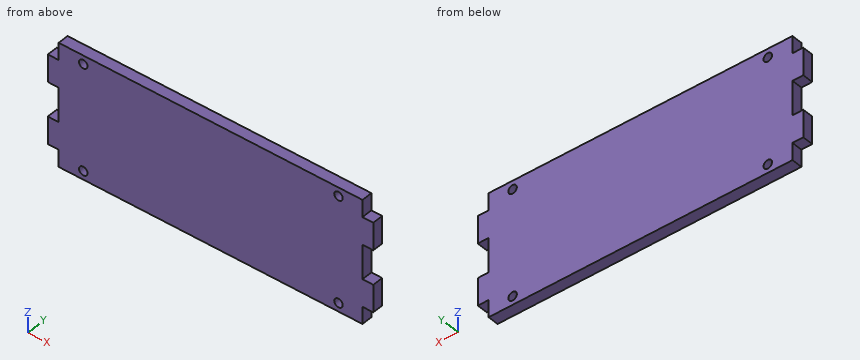
```python
from build123d import *

# Parameters (mm, degrees)
SKETCH1_R           = 1.25
BOSS_EXTRUDE1_DEPTH = 3.18


with BuildPart() as part:
    # Sketch1 → Boss-Extrude1 (new body)
    with BuildSketch(Plane(origin=(0, 0, 0), x_dir=(1, 0, 0), z_dir=(0, 1, 0))):
        Polygon((-47.930848892, -13), (-44.750848892, -13), (-44.750848892, -18), (-40, -18), (-37.5, -18), (37.5, -18), (40, -18), (44.539151108, -18), (44.539151108, -13), (47.719151108, -13), (47.719151108, -5), (44.539151108, -5), (44.539151108, 5), (47.719151108, 5), (47.719151108, 13), (44.539151108, 13), (44.539151108, 18), (40, 18), (37.5, 18), (-37.5, 18), (-40, 18), (-44.750848892, 18), (-44.750848892, 13), (-47.930848892, 13), (-47.930848892, 5), (-44.750848892, 5), (-44.750848892, -5), (-47.930848892, -5), align=None)
        with Locations(Location((37.5, 15.5, 0), (0, 0, 90))):
            Circle(SKETCH1_R, mode=Mode.SUBTRACT)
        with Locations(Location((37.5, -15.5, 0), (0, 0, 90))):
            Circle(SKETCH1_R, mode=Mode.SUBTRACT)
        with Locations(Location((-37.5, -15.5, 0), (0, 0, 90))):
            Circle(SKETCH1_R, mode=Mode.SUBTRACT)
        with Locations(Location((-37.5, 15.5, 0), (0, 0, 90))):
            Circle(SKETCH1_R, mode=Mode.SUBTRACT)
    extrude(amount=BOSS_EXTRUDE1_DEPTH)


solid = part.part
```
The listing builds one solid part. Answer for the finished solid, in the listing's coordinates (mm). Give positions to 0.01 mm unless a question says otherwise; leave off trailing zeros. Loops run counter-clockwise (first coordinate to the right, second up) from the corner with the lowest first, then second, coordinate; pieces in that order, holes last. Notation, with made-up numbers: M 68,41.25 L 96,41.25 A26 cw 96,55.25 Z; hole C 38,-35 d3. An arc over 180 degrees is marked long. One line per item, written item: value.
Q1. A cutting plane is placed at A-A on x = 37.5. Determine the outline of the cut face in (y, z).
Working result:
outline: M 0,-18 L 3.18,-18 L 3.18,-16.75 L 0,-16.75 Z; M 0,-14.25 L 3.18,-14.25 L 3.18,14.25 L 0,14.25 Z; M 0,16.75 L 3.18,16.75 L 3.18,18 L 0,18 Z
Q2. Find the intervals of material crossed by line 1 (X direction, y = 1.55, z = 15.5); line 2 (Z direction, x = 37.5, y = 1.9); line 3 (Z direction, x = 37, y = 0.85), in increasing order. Write a range as from..to.
Working result:
line 1: x = -44.75..-38.75, -36.25..36.25, 38.75..44.54
line 2: z = -18..-16.75, -14.25..14.25, 16.75..18
line 3: z = -18..-16.65, -14.35..14.35, 16.65..18
Q3. A cutting plane is placed at B-B on z = -15.5. Determine the outline of the cut face in (x, y), then the cut area to 3 significant figures.
Working result:
outline: M -44.75,0 L -38.75,0 L -38.75,3.18 L -44.75,3.18 Z; M -36.25,0 L 36.25,0 L 36.25,3.18 L -36.25,3.18 Z; M 38.75,0 L 44.54,0 L 44.54,3.18 L 38.75,3.18 Z
area: 268 mm^2
Q4. A flat-ended cylindrical pin translates along its axis: P1, Ø1, axis at x = -46, y = 1.5, coming from the +Z side. Find the tip coordinate at first contact, or state that the pin passes through.
Working result:
P1: stops at z = 13
Q5. A cutting plane is placed at C-C on y = 1.9. Determine the outline of the cut face in (x, z), then the cut area to 3 significant figures.
Working result:
outline: M -47.93,-13 L -44.75,-13 L -44.75,-18 L 44.54,-18 L 44.54,-13 L 47.72,-13 L 47.72,-5 L 44.54,-5 L 44.54,5 L 47.72,5 L 47.72,13 L 44.54,13 L 44.54,18 L -44.75,18 L -44.75,13 L -47.93,13 L -47.93,5 L -44.75,5 L -44.75,-5 L -47.93,-5 Z; hole C -37.5,-15.5 d2.5; hole C -37.5,15.5 d2.5; hole C 37.5,-15.5 d2.5; hole C 37.5,15.5 d2.5
area: 3,300 mm^2
